Can you work these out from the drawing? Everything is in mm from the part's minimum corner. A direction names the side the tool comes from. Give positions to 0.01 mm unless a question says otherwise; leave off trailing zeros. Order: outer loops, then holes, each group sorted by start corner. A loop starts at its lowest first (then second) coordinate and runs counter-clockwise, first axis right, second up. Notation, with made-up numbers: (74, 4.5) - (104, 4.5) arc R19 cw to (104, 38.5) - close; hole circle Ø1 at (72, 68). An arc over 180 degrees is marked (long way). Answer as a JSON object with one key per item and string values.
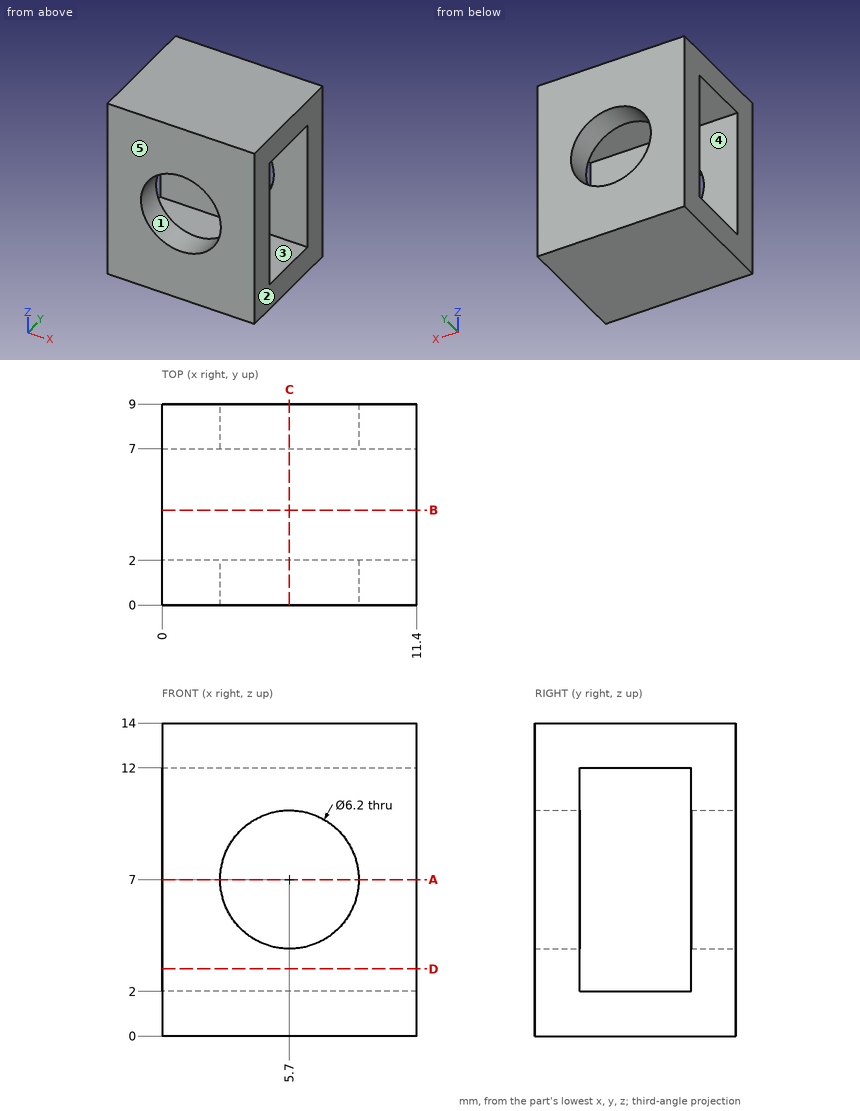
Q1. We'd pull the mould along X, two halves only. Please class the marked faces 1, 2 and 3: released by +X, released by -X, zero draft, split by the parting line, or undercut.
Recorded:
{"face 1": "undercut", "face 2": "released by +X", "face 3": "zero draft"}
Q2. If we section it at B-B, the plane y = 4.25: Please give me the cut outline in (x, z), then the cut area to 3 significant figures.
Recorded:
{"outline": "(0, 0) - (11.4, 0) - (11.4, 2) - (0, 2) - close; (0, 12) - (11.4, 12) - (11.4, 14) - (0, 14) - close", "area": "45.6 mm^2"}
Q3. Which directions (+Z, -Z, +X, -X, +Y, -Y) give clear straight access to the entire face, cutting with the end or side of a thin tool? Please do the marked faces 4 and 5.
Recorded:
{"face 4": "+X, -X", "face 5": "+Z, -Z, +X, -X, -Y"}
Q4. If we section it at D-D, the plane z = 3: Please give me the cut outline in (x, y).
Recorded:
{"outline": "(0, 0) - (11.4, 0) - (11.4, 2) - (0, 2) - close; (0, 7) - (11.4, 7) - (11.4, 9) - (0, 9) - close"}
Q5. If we section it at C-C, the plane x = 5.7: Please give me the cut outline in (y, z).
Recorded:
{"outline": "(0, 0) - (9, 0) - (9, 3.9) - (7, 3.9) - (7, 2) - (2, 2) - (2, 3.9) - (0, 3.9) - close; (0, 10.1) - (2, 10.1) - (2, 12) - (7, 12) - (7, 10.1) - (9, 10.1) - (9, 14) - (0, 14) - close"}
Q6. I need wall thicknesses on L1, parallel to X at y = 1, z = 7; L2, parallel to Z at x = 5.7, y = 7.65; L3, parallel to Z at x = 4.5, y = 3.5. Which ranges of each line are inside material? Lowest first, please.
Recorded:
{"L1": "x = 0 to 2.6, 8.8 to 11.4", "L2": "z = 0 to 3.9, 10.1 to 14", "L3": "z = 0 to 2, 12 to 14"}
Q7. If we section it at A-A, the plane z = 7: Please give me the cut outline in (x, y).
Recorded:
{"outline": "(0, 0) - (2.6, 0) - (2.6, 2) - (0, 2) - close; (0, 7) - (2.6, 7) - (2.6, 9) - (0, 9) - close; (8.8, 0) - (11.4, 0) - (11.4, 2) - (8.8, 2) - close; (8.8, 7) - (11.4, 7) - (11.4, 9) - (8.8, 9) - close"}
